Check sheet for the drawn part. Datum: minimum x, y, z corner. Units: mm. A direction names the side the tool comes from. Give positions to 0.01 mm unless a question says otherwise; leave off trailing zeros. Order: outer loops, then holes, each group sorted by start corner. A loop starts at its lowest first (then second) coordinate and runs counter-clockwise, first axis right, second up. Notation, with made-up numbers: M 68.25,41 L 127.25,41 A22 ccw 127.25,49 Z; hole C 82,7 d2. An arc over 180 degrees is marked long. Put each result on its own line as item: value. Start each with the question number.
Q1. Section check C-C on z = 27.5. Record the cut outline in (x, y), then the cut area to 3 significant figures.
Q2. Material ranges on L1, parallel to X at y = 120, z = 9; L2, parallel to Z at x = 50.5, y = 109.5; L3, parallel to Y at x = 95.5, z = 19.5 (1 decimal), recorded low to high.
Q3. Mould release check, pull along X, two halves, no side actions. Record for the marked faces 3, 4 and 5: +X half, -X half, draft (parallel to the pull), parting line (faces both ways), or undercut.
Q4. Section check B-B on z = 17. Record the cut outline in (x, y) (1 decimal), then the cut area to 3 significant figures.
Q5. Access from +Z, -Z, +X, -X, +Y, -Y to the whole of each face (thin tool, end or side, straight path). Record for the marked faces 1 and 2.
Q6. Section check D-D on y = 100.5. Record the cut outline in (x, z) (1 decimal), then the cut area to 3 significant figures.
Q7. Section check A-A on x = 20. Record the cut outline in (y, z) (1 decimal), then the cut area to 3 significant figures.
Q8. Go/stop test with flat-tipped pins: pin 1 (12 mm diameter, centred on x = 95, y = 90.5, fed in from -Z); pin 2 (3 mm diameter, centred on y = 131.37, z = 4.13, fed in from +X); pin 3 (15 mm diameter, centred on x = 67, y = 19.5, fed in from -Z). Record where each tip stops, or that it passes through.
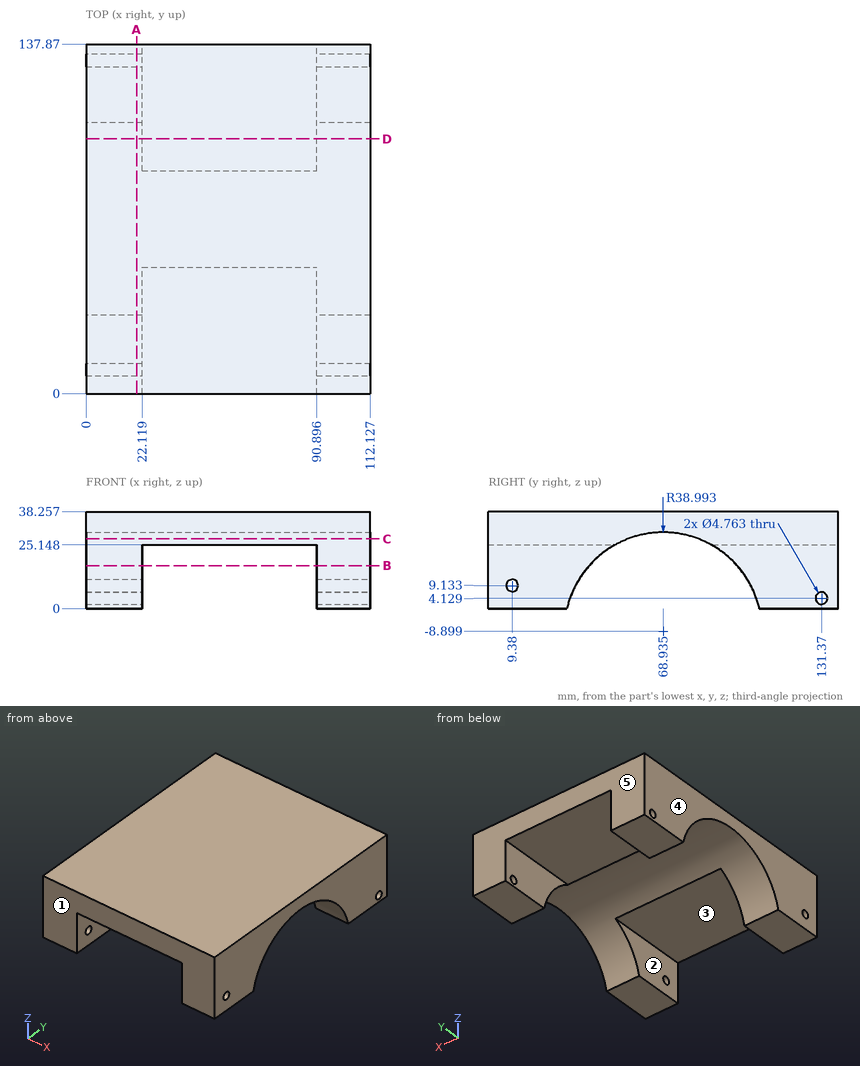
Results found:
1. outline: M 0,0 L 112.13,0 L 112.13,54.95 L 0,54.95 Z; M 0,82.92 L 112.13,82.92 L 112.13,137.87 L 0,137.87 Z
1. area: 12,300 mm^2
2. L1: x = 0 to 22.12, 90.9 to 112.13
2. L2: z = 25.15 to 38.26
2. L3: y = 0 to 42.2, 95.7 to 137.9
3. face 3: undercut
3. face 4: -X half
3. face 5: draft
4. outline: M 0,0 L 22.1,0 L 22.1,39.8 L 0,39.8 Z; M 0,98.1 L 22.1,98.1 L 22.1,137.9 L 0,137.9 Z; M 90.9,0 L 112.1,0 L 112.1,39.8 L 90.9,39.8 Z; M 90.9,98.1 L 112.1,98.1 L 112.1,137.9 L 90.9,137.9 Z
4. area: 3,450 mm^2
5. face 1: +Z, -Z, +X, -X, -Y
5. face 2: -Z, +Y, -Y
6. outline: M 0,14 L 22.1,14 L 22.1,25.1 L 90.9,25.1 L 90.9,14 L 112.1,14 L 112.1,38.3 L 0,38.3 Z
6. area: 1,950 mm^2
7. outline: M 0,0 L 31,0 A39 cw 106.9,0 L 137.9,0 L 137.9,38.3 L 0,38.3 Z; hole C 9.4,9.1 d4.8; hole C 131.4,4.1 d4.8
7. area: 3,540 mm^2
8. pin 1: stops at z = 18.68
8. pin 2: passes through
8. pin 3: stops at z = 25.15
